The listing builds one solid part. Answer for the finished solid, in the listing's coordinates (mm). Face numbers are marked on the shaded views. A direction names the side the tool comes from. Round coordinates to 2 decimals unless told otherwise and drop trailing zeros. Write each loop counter-clockwise with the first axis right and the second up, starting at its lowest first coordinate (ties: lowest second). Pieces come first, ordered by that corner, then holes. Notation, with made-up numbers: (35.5, 80) - (93.5, 80) arc R7 ccw to (93.5, 84) - close; hole circle Ø1 at (16, 3). An arc over 180 degrees is marked (long way). Answer as CSV lines item,"result". Start each with the question number.
Item 1: Straight lines are drawn through the part: line 1 along Z through (x, y) = (34, 1.35); line 2 along Y through (x, z) = (1.2, 30); line 3 along Y through (x, z) = (11, 34.5). For each, find the intervals that lie inside material, in ascending order. Write a range as [from, to].
Item 2: A cutting plane is placed at D-D on z = 5. Determine the outline of the cut face in (x, y).
Item 3: A cutting plane is placed at A-A on y = 34. Determine the outline of the cut face in (x, z).
Item 4: Flat-ended cylindrical pins translate along their axes: pin 1 (7 mm diameter, centred on x = 34, z = 30, fed in from +Y); pin 2 (18 mm diameter, centred on y = 22, z = 12.5, fed in from +X). Find the tip coordinate at first contact, or state that the pin passes through.
Item 5: A cutting plane is placed at B-B on z = 30. Determine the outline of the cut face in (x, y).
Item 6: Which of the six approach directions +Z, -Z, +X, -X, +Y, -Y give full straight-line access (tool end or side, diameter ignored) to the marked faces 1 and 2?
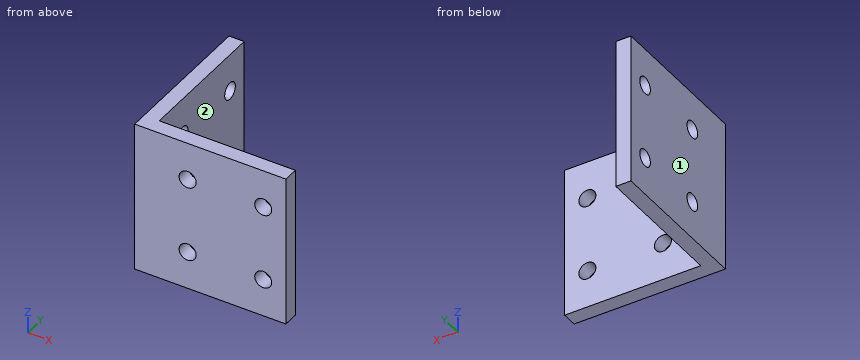
```python
from build123d import *

# Parameters (mm, degrees)
EXTRUDE_1_DEPTH       = 40
HOLE_WIZARD_M41_D     = 4.5
HOLE_WIZARD_M41_DEPTH = 5
HOLE_WIZARD_M41_TIP   = 1.351936393
HOLE_WIZARD_M42_D     = 4.5
HOLE_WIZARD_M42_DEPTH = 5
HOLE_WIZARD_M42_TIP   = 1.351936393


with BuildPart() as part:
    # Эскиз1 → Бобышка-Вытянуть1 (new body)
    with BuildSketch(Plane.XY):
        Polygon((0, 0), (0, 40), (4, 40), (4, 4), (40, 4), (40, 0), align=None)
    extrude(amount=EXTRUDE_1_DEPTH)

    # Отверстие с зазором M41
    with Locations(Plane(origin=(0, 4, 0), x_dir=(-1, 0, 0), z_dir=(0, 1, 0))):
        with Locations((-34, 10), (-14, 10), (-34, 30), (-14, 30)):
            Hole(HOLE_WIZARD_M41_D / 2, depth=HOLE_WIZARD_M41_DEPTH)
            with Locations((0, 0, -(HOLE_WIZARD_M41_DEPTH + HOLE_WIZARD_M41_TIP / 2))):  # 118° drill point
                Cone(0, HOLE_WIZARD_M41_D / 2, HOLE_WIZARD_M41_TIP, mode=Mode.SUBTRACT)

    # Отверстие с зазором M42
    with Locations(Plane(origin=(4, 0, 0), x_dir=(0, 0, -1), z_dir=(1, 0, 0))):
        with Locations((-10, 34), (-30, 34), (-10, 14), (-30, 14)):
            Hole(HOLE_WIZARD_M42_D / 2, depth=HOLE_WIZARD_M42_DEPTH)
            with Locations((0, 0, -(HOLE_WIZARD_M42_DEPTH + HOLE_WIZARD_M42_TIP / 2))):  # 118° drill point
                Cone(0, HOLE_WIZARD_M42_D / 2, HOLE_WIZARD_M42_TIP, mode=Mode.SUBTRACT)


solid = part.part
```
Geometry says:
1,line 1,"z = [0, 7.75], [12.25, 27.75], [32.25, 40]"
1,line 2,"y = [0, 11.75], [16.25, 31.75], [36.25, 40]"
1,line 3,"y = [0, 4]"
2,outline,"(0, 0) - (40, 0) - (40, 4) - (4, 4) - (4, 40) - (0, 40) - close"
3,outline,"(0, 0) - (4, 0) - (4, 7.75) - (0, 7.75) - close; (0, 12.25) - (4, 12.25) - (4, 27.75) - (0, 27.75) - close; (0, 32.25) - (4, 32.25) - (4, 40) - (0, 40) - close"
4,pin 1,"stops at y = 4"
4,pin 2,"stops at x = 4"
5,outline,"(0, 0) - (11.75, 0) - (11.75, 4) - (4, 4) - (4, 11.75) - (0, 11.75) - close; (0, 16.25) - (4, 16.25) - (4, 31.75) - (0, 31.75) - close; (0, 36.25) - (4, 36.25) - (4, 40) - (0, 40) - close; (16.25, 0) - (31.75, 0) - (31.75, 4) - (16.25, 4) - close; (36.25, 0) - (40, 0) - (40, 4) - (36.25, 4) - close"
6,face 1,"+Z, -Z, -X, +Y, -Y"
6,face 2,"+Z, -Z, +X, +Y"
